For this review, use the dimensioned drawing (mm, ordinates from the lowest corner) and the shaded views. Round coordinates to 2 decimals unless told otherwise and drop trailing zeros. Order: outer loops, then holes, each group sorted by start corner. A loop starts at its lowest first (then second) coordinate and runs counter-clockwise, first axis right, second up. Notation, with made-up numbers: M 72.25,-35 L 89.25,-35 A24 ccw 89.25,-7 Z; hole C -32.75,62 d11. An arc over 180 degrees is marked long. Put each result on its own line as item: value.
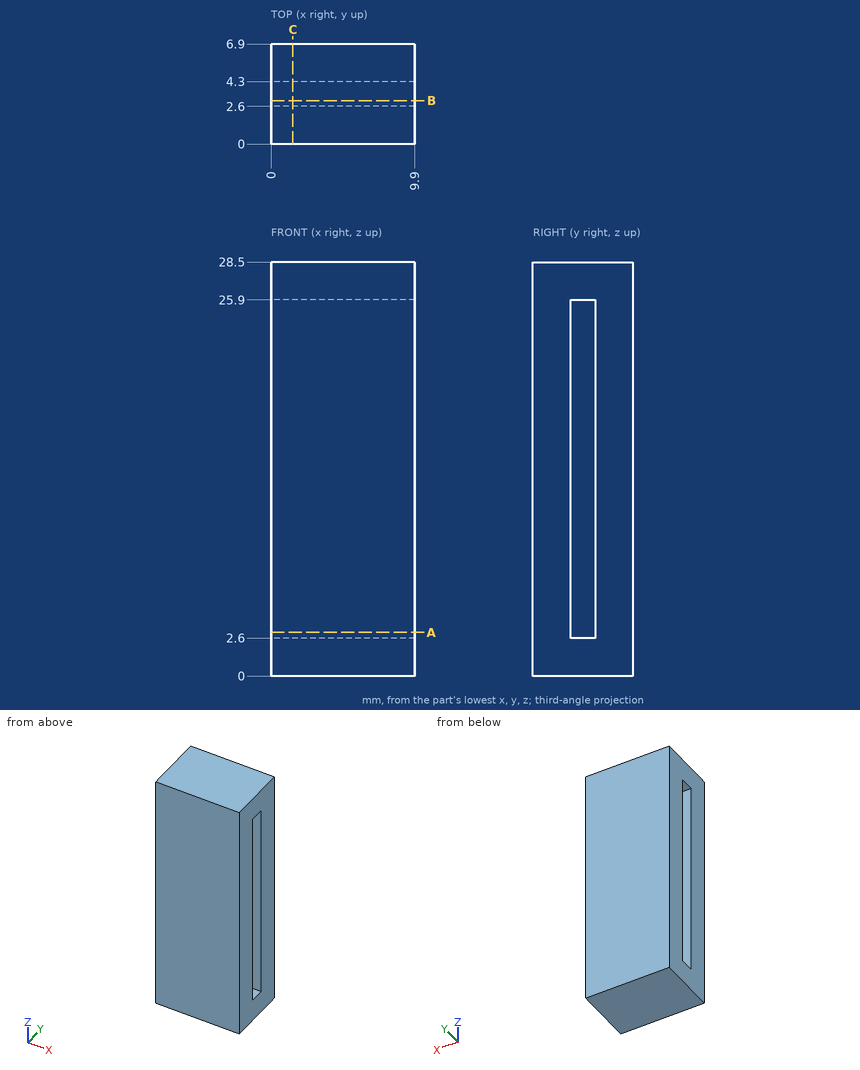
(1) Add section A-A on z = 3. Give the boundary of the cut face in (x, y).
A:
outline: M 0,0 L 9.9,0 L 9.9,2.6 L 0,2.6 Z; M 0,4.3 L 9.9,4.3 L 9.9,6.9 L 0,6.9 Z
(2) Add section B-B on y = 3. Give the boundary of the cut face in (x, z).
A:
outline: M 0,0 L 9.9,0 L 9.9,2.6 L 0,2.6 Z; M 0,25.9 L 9.9,25.9 L 9.9,28.5 L 0,28.5 Z
(3) Add section C-C on x = 1.5. Give the boundary of the cut face in (y, z).
A:
outline: M 0,0 L 6.9,0 L 6.9,28.5 L 0,28.5 Z; hole M 2.6,2.6 L 4.3,2.6 L 4.3,25.9 L 2.6,25.9 Z
(4) To check wall thickness, follow L1, parallel to Y at x = 3.5, z = 6; L2, parallel to Z at x = 3.25, y = 2.75. State the ranges of each line that lie inside material, in increasing order.
A:
L1: y = 0 to 2.6, 4.3 to 6.9
L2: z = 0 to 2.6, 25.9 to 28.5
